Verification items for the finished model (mm, model axes). Face numbers are marked on the shaded views. A direction names the side the tool comes from. Give positions to 0.01 mm unless a question says otherwise; leave off trailing zeros. Loops run counter-clockwise (first coordinate to the right, second up) from the corner with the lowest first, then second, coordinate; pieces in that order, holes last. Notation, with made-up numbers: M 1.25,-31 L 38.25,-31 A18 ccw 38.25,-21 Z; hole C -28.75,65 d2. An arc over 180 degrees is marked long. Use a Markdown table: item, result.
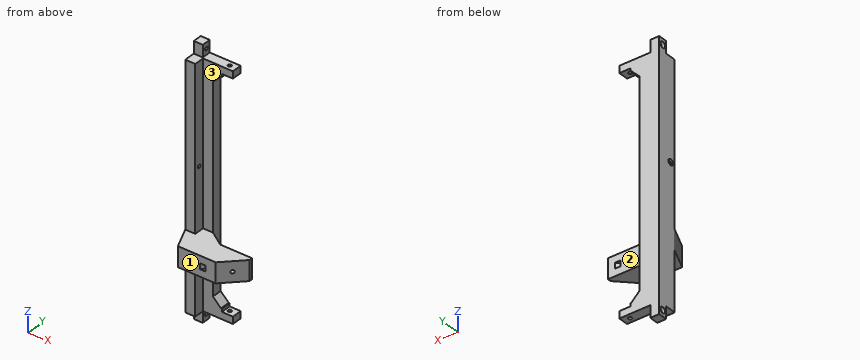
from build123d import *

# Parameters (mm, degrees)
BOSS_EXTRUDE1_DEPTH = 240
BOSS_EXTRUDE3_DEPTH = 10
SKETCH5_R           = 1.75
CUT_EXTRUDE1_DEPTH  = 243.69322199
SKETCH6_W           = 7
SKETCH6_H           = 12
CUT_EXTRUDE2_DEPTH  = 11
SKETCH7_W           = 20
SKETCH7_H           = 22.38
BOSS_EXTRUDE4_DEPTH = 57.02
BOSS_EXTRUDE5_DEPTH = 20
CUT_EXTRUDE3_DEPTH  = 20
SKETCH14_W          = 9
SKETCH14_H          = 9
BOSS_EXTRUDE6_DEPTH = 12
SKETCH15_W          = 9
SKETCH15_H          = 9
BOSS_EXTRUDE7_DEPTH = 12
SKETCH18_R          = 1.75
CUT_EXTRUDE10_DEPTH = 9
SKETCH19_R          = 3
CUT_EXTRUDE11_DEPTH = 3.1
SKETCH20_R          = 1.75
CUT_EXTRUDE12_DEPTH = 10
CUT_EXTRUDE13_DEPTH = 2.1
SKETCH22_R          = 1.75
CUT_EXTRUDE14_DEPTH = 15
SKETCH24_W          = 4
SKETCH24_H          = 5.7
CUT_EXTRUDE15_DEPTH = 260.337896961


with BuildPart() as part:
    # Sketch1 → Boss-Extrude1 (new body)
    with BuildSketch(Plane.XY):
        Polygon((-10, 0), (0, 0), (0, 10), (10, 10), (10, 20), (-10, 20), align=None)
    extrude(amount=BOSS_EXTRUDE1_DEPTH)

    # Sketch4 → Boss-Extrude3 (add)
    with BuildSketch(Plane(origin=(0, 20, 0), x_dir=(1, 0, 0), z_dir=(0, 1, 0))):
        Polygon((10, 0), (30, 0), (30, -10), (18, -10), (10, -18), align=None)
    boss_extrude3 = extrude(amount=-BOSS_EXTRUDE3_DEPTH)

    # Sketch5 → Cut-Extrude1 (cut, through all)
    with BuildSketch(Plane(origin=(0, 0, 0), x_dir=(-1, 0, 0), z_dir=(0, 0, -1))):
        with Locations((-23, 15)):
            Circle(SKETCH5_R)
    cut_extrude1 = extrude(amount=-CUT_EXTRUDE1_DEPTH, mode=Mode.SUBTRACT)

    # Sketch6 → Cut-Extrude2 (cut)
    with BuildSketch(Plane(origin=(30, 0, 0), x_dir=(0, 0, -1), z_dir=(1, 0, 0))):
        with Locations((-10.5, 15)):
            Rectangle(SKETCH6_W, SKETCH6_H)
    cut_extrude2 = extrude(amount=-CUT_EXTRUDE2_DEPTH, mode=Mode.SUBTRACT)

    # Mirror1: Boss-Extrude3, Cut-Extrude1, Cut-Extrude2 across plane
    add(boss_extrude3.mirror(Plane(origin=(0, 0, 120), x_dir=(1, 0, 0), z_dir=(0, 0, -1))))
    add(cut_extrude1.mirror(Plane(origin=(0, 0, 120), x_dir=(1, 0, 0), z_dir=(0, 0, -1))), mode=Mode.SUBTRACT)
    add(cut_extrude2.mirror(Plane(origin=(0, 0, 120), x_dir=(1, 0, 0), z_dir=(0, 0, -1))), mode=Mode.SUBTRACT)



with BuildPart() as body_2:
    # Sketch7 → Boss-Extrude4 (new body)
    with BuildSketch(Plane(origin=(0, 0, 0), x_dir=(0, 0, -1), z_dir=(1, 0, 0))):
        with Locations((-68.66, -11.19)):
            Rectangle(SKETCH7_W, SKETCH7_H)
    extrude(amount=BOSS_EXTRUDE4_DEPTH)


with BuildPart() as part_1:
    add(part.part)

    add(body_2.part)  # Boss-Extrude5 merges body 2
    # Sketch9 → Boss-Extrude5 (add)
    with BuildSketch(Plane(origin=(0, 0, 58.66), x_dir=(-1, 0, 0), z_dir=(0, 0, -1))):
        Polygon((-10, 10), (10, 10), (10, 0), (0, -22.38), (-25, -22.38), (-25, 0), align=None)
    extrude(amount=-BOSS_EXTRUDE5_DEPTH)

    # Sketch10 → Cut-Extrude3 (cut)
    with BuildSketch(Plane(origin=(0, 0, 58.66), x_dir=(-1, 0, 0), z_dir=(0, 0, -1))):
        Polygon((-31.667249158, -28.601477466), (-43.135001652, -40.069229961), (-74.531570141, -8.672661471), (-63.063817647, 2.795091023), align=None)
    extrude(amount=-CUT_EXTRUDE3_DEPTH, mode=Mode.SUBTRACT)

    # Sketch14 → Boss-Extrude6 (add)
    with BuildSketch(Plane(origin=(0, 0, 0), x_dir=(-1, 0, 0), z_dir=(0, 0, -1))):
        with Locations((5.5, 15.5)):
            Rectangle(SKETCH14_W, SKETCH14_H)
    extrude(amount=BOSS_EXTRUDE6_DEPTH)

    # Sketch15 → Boss-Extrude7 (add)
    with BuildSketch(Plane.XY.offset(240)):
        with Locations((-5.5, 15.5)):
            Rectangle(SKETCH15_W, SKETCH15_H)
    extrude(amount=BOSS_EXTRUDE7_DEPTH)

    # Sketch18 → Cut-Extrude10 (cut)
    with BuildSketch(Plane.ZY.offset(10)):
        with Locations(Location((-6, 15.5, 0), (0, 0, 270))):
            Circle(SKETCH18_R)
        with Locations(Location((246, 15.5, 0), (0, 0, 270))):
            Circle(SKETCH18_R)
    extrude(amount=-CUT_EXTRUDE10_DEPTH, mode=Mode.SUBTRACT)

    # Sketch19 → Cut-Extrude11 (cut)
    with BuildSketch(Plane.ZY.offset(10)):
        with Locations(Location((-6, 15.5, 0), (0, 0, 270))):
            Circle(SKETCH19_R)
        with Locations(Location((246, 15.5, 0), (0, 0, 270))):
            Circle(SKETCH19_R)
    extrude(amount=-CUT_EXTRUDE11_DEPTH, mode=Mode.SUBTRACT)

    # Sketch20 → Cut-Extrude12 (cut)
    with BuildSketch(Plane.ZY.offset(10)):
        with Locations(Location((140, 5, 0), (0, 0, 270))):
            Circle(SKETCH20_R)
    extrude(amount=-CUT_EXTRUDE12_DEPTH, mode=Mode.SUBTRACT)

    # Sketch21 → Cut-Extrude13 (cut)
    with BuildSketch(Plane.ZY.offset(10)):
        Polygon((141.645448267, 2.15), (143.290896534, 5), (141.645448267, 7.85), (138.354551733, 7.85), (136.709103466, 5), (138.354551733, 2.15), align=None)
    extrude(amount=-CUT_EXTRUDE13_DEPTH, mode=Mode.SUBTRACT)

    # Sketch22 → Cut-Extrude14 (cut)
    with BuildSketch(Plane(origin=(30.134363312, -30.134363312, 0), x_dir=(0, 0, -1), z_dir=(0.7071067811865474, -0.7071067811865477, 0))):
        with Locations(Location((-68.66, 24.452032037, 0), (0, 0, 90))):
            Circle(SKETCH22_R)
    extrude(amount=-CUT_EXTRUDE14_DEPTH, mode=Mode.SUBTRACT)

    # Sketch24 → Cut-Extrude15 (cut, through all)
    with BuildSketch(Plane(origin=(0, 0, 0), x_dir=(0.7071067811865477, -0.7071067811865475, 0), z_dir=(0.7071067811865475, 0.7071067811865477, 0))):
        with Locations((33.319228663, -68.66)):
            Rectangle(SKETCH24_W, SKETCH24_H)
    extrude(amount=CUT_EXTRUDE15_DEPTH, mode=Mode.SUBTRACT)


solid = part_1.part
(1) Cross-section at A-A on y = -19. Record the cut outline in (x, z), then the cut area to 3 significant figures.
Results below:
| item | result |
|---|---|
| outline | M -1.51,58.66 L 41.27,58.66 L 41.27,78.66 L -1.51,78.66 Z; hole M 25.29,65.81 L 30.95,65.81 L 30.95,71.51 L 25.29,71.51 Z |
| area | 823 mm^2 |
(2) Cross-section at C-C on y = -9. State how many separate pieces and enclosed holes the cut face has, then the cut area to 3 significant figures.
Results below:
| item | result |
|---|---|
| separate pieces | 1 |
| enclosed holes | 2 |
| area | 1,100 mm^2 |
(3) Gauge pin test, flat ends, axial feed: P1, Ø4.5, axis at x = -5.5, z = -8.5, coming from the -Y side; P2, Ø3, axis at x = -6.5, z = 21, coming from the -Y side; P3, Ø12, axis at x = -3, y = -16, coming from the +Z side; P4, Ø2, axis at x = 23, y = 15, coming from the +Z side. Record the tip position at first contact, or that the pin passes through.
Results below:
| item | result |
|---|---|
| P1 | y = 11 |
| P2 | y = 0 |
| P3 | z = 78.66 |
| P4 | through |
(4) Cross-section at B-B on z = 147. Record the cut outline in (x, y), then the cut area to 3 significant figures.
Results below:
| item | result |
|---|---|
| outline | M -10,0 L 0,0 L 0,10 L 10,10 L 10,20 L -10,20 Z |
| area | 300 mm^2 |
(5) Material ranges on line 1 (Z direction, x = -5.05, y = 15.5); line 2 (Z direction, x = -8.55, y = 15.5); line 3 (X direction, y = 15, z = 235), recorded low to high.
Results below:
| item | result |
|---|---|
| line 1 | -12 to -7.75, -4.25 to 244.25, 247.75 to 252 |
| line 2 | -12 to -9, -3 to 243, 249 to 252 |
| line 3 | -10 to 21.25, 24.75 to 30 |
(6) Set-up check for the marked faces 1, 2 and 3: record each of +Z, -Z, +X, -X, +Y, -Y from which the full face is reachable in a straight line by a thin tool's end or side.
Results below:
| item | result |
|---|---|
| face 1 | +Z, -Z, +X, -X, -Y |
| face 2 | +Z, -Z, +X, +Y |
| face 3 | +Z, +X, -Y |
